```python
from build123d import *

# Parameters (mm, degrees)
SKETCH_1_W          = 42
SKETCH_1_H          = 76.3
EXTRUDE_1_DEPTH     = 20.5
FILLET_1_R          = 8
SHELL_1_T           = 2.3
CUT_EXTRUDE_START   = 2.2
SKETCH_3_W          = 37.8
SKETCH_3_H          = 71.7
CUT_EXTRUDE_1_DEPTH = 19.3
SKETCH_1_3_R        = 1.5
CUT_EXTRUDE_2_DEPTH = 21.5
SKETCH_4_W          = 1
SKETCH_4_H          = 76.3
EXTRUDE_2_DEPTH     = 20.5
CHAMFER1_SIZE       = 1.3


with BuildPart() as part:
    # Эскиз1 → Бобышка-Вытянуть1 (new body)
    with BuildSketch(Plane(origin=(0, 0, 0), x_dir=(1, 0, 0), z_dir=(0, 1, 0))):
        Rectangle(SKETCH_1_W, SKETCH_1_H)
    extrude(amount=EXTRUDE_1_DEPTH)

    # Скругление1
    fillet_1_edges = [part.edges().sort_by_distance(p)[0] for p in [
        (-21, 20.5, 0),
        (21, 20.5, 0),
    ]]
    fillet(fillet_1_edges, radius=FILLET_1_R)

    # Оболочка1 (no face opened: a closed hollow body)
    add(offset(amount=-SHELL_1_T, mode=Mode.PRIVATE), mode=Mode.SUBTRACT)

    # Эскиз3 → Вырез-Вытянуть1 (cut, through all)
    with BuildSketch(Plane(origin=(0, 0, 0), x_dir=(1, 0, 0), z_dir=(0, 1, 0)).offset(CUT_EXTRUDE_START)):
        Rectangle(SKETCH_3_W, SKETCH_3_H)
    extrude(amount=CUT_EXTRUDE_1_DEPTH, mode=Mode.SUBTRACT)

    # Эскиз1<3> → Вырез-Вытянуть2 (cut, through all)
    with BuildSketch(Plane(origin=(0, 0, 0), x_dir=(1, 0, 0), z_dir=(0, 1, 0))):
        with Locations((-10.5, 0)):
            Circle(SKETCH_1_3_R)
        with Locations((10.5, 0)):
            Circle(SKETCH_1_3_R)
    extrude(amount=CUT_EXTRUDE_2_DEPTH, mode=Mode.SUBTRACT)

    # Эскиз4 → Бобышка-Вытянуть2 (add)
    with BuildSketch(Plane(origin=(0, 0, 0), x_dir=(1, 0, 0), z_dir=(0, 1, 0))):
        Rectangle(SKETCH_4_W, SKETCH_4_H)
    extrude(amount=EXTRUDE_2_DEPTH)

    # Chamfer1
    chamfer1_edges = [part.edges().sort_by_distance(p)[0] for p in [
        (9, 2.2, 0),
        (-12, 2.2, 0),
    ]]
    chamfer(chamfer1_edges, length=CHAMFER1_SIZE)


solid = part.part
```
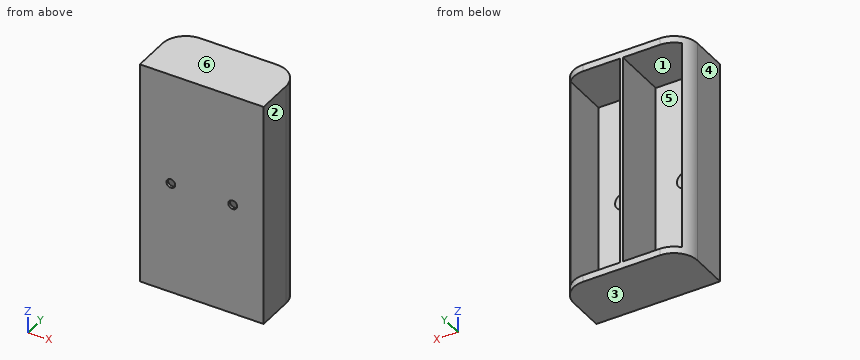
For this review, take the finished solid that the model builds, in its own axes (mm). Face numbers are marked on the shaded views. A direction names the side the tool comes from. Coordinates: 2 decimals unless noted, no trailing zeros. Write each loop counter-clockwise with the first axis right and the second up, starting at its lowest first coordinate (ties: lowest second). Pieces come first, ordered by that corner, then holes.
(1) The part is to be moulded in two halves that separate along Z. For the marked faces 3, 4, 5 and 6, say which applies: +Z half, -Z half, draft (parallel to the pull), parting line (faces both ways), or undercut.
(2) Add section C-C on x = 5.5. Give the boundary of the cut face in (y, z), then the cut area to 3 significant figures.
(3) Add section B-B on y = 5.25. Give the boundary of the cut face in (x, z).
(4) Tool access review of the marked faces 1 and 2: name each direction out of +Z, -Z, +X, -X, +Y, -Y from which nothing blocks a thin tool from reaching the whole face with its end or side.
(5) For pin 1 Ø8 at (x, z) = (7.5, 6.5) entering from -Y; pin 2 Ø4 at (y, z) = (16, 20.5) entering from -X; pin 3 Ø9 at (x, z) = (6.5, 15) entering from +Y; pin 4 Ø1 at (y, z) = (16, -6.5) entering from -X, all flat-tipped, find the tip position at first contact; note any pin that passes through.
(6) Wall thickness on probe 1 along X at (y, z) = (2.25, 30.5); probe 2 along X at (y, z) = (0.2, 0); probe 3 along Z at (x, y) = (10.5, 0.45): over which ranges is each line inside the solid? List them lowest first.
(7) Add section D-D on z = -19. Give the boundary of the cut face in (x, y).
(8) Add section A-A on x = 10.5. Give the boundary of the cut face in (y, z), then the cut area to 3 significant figures.
Answer sheet:
1. face 3: -Z half
1. face 4: draft
1. face 5: undercut
1. face 6: +Z half
2. outline: (0, -38.15) - (20.5, -38.15) - (20.5, -35.85) - (2.2, -35.85) - (2.2, 35.85) - (20.5, 35.85) - (20.5, 38.15) - (0, 38.15) - close
2. area: 252 mm2
3. outline: (-21, -38.15) - (21, -38.15) - (21, 38.15) - (-21, 38.15) - close; hole (-18.9, -35.85) - (-0.5, -35.85) - (-0.5, 35.85) - (-18.9, 35.85) - close; hole (0.5, -35.85) - (18.9, -35.85) - (18.9, 35.85) - (0.5, 35.85) - close
4. face 1: +Y
4. face 2: +Z, -Z, +X, +Y, -Y
5. pin 1: stops at y = 0
5. pin 2: stops at x = -20.86
5. pin 3: stops at y = 2.2
5. pin 4: stops at x = -20.42
6. probe 1: x = -21 to -18.9, -0.5 to 0.5, 18.9 to 21
6. probe 2: x = -21 to -12, -9 to 9, 12 to 21
6. probe 3: z = -38.15 to -1.5, 1.5 to 38.15
7. outline: (-21, 0) - (21, 0) - (21, 12.5) arc R8 ccw to (18.9, 17.9) - (18.9, 2.2) - (0.5, 2.2) - (0.5, 20.5) - (-0.5, 20.5) - (-0.5, 2.2) - (-18.9, 2.2) - (-18.9, 17.9) arc R8 ccw to (-21, 12.5) - close
8. outline: (0, -38.15) - (20.5, -38.15) - (20.5, -35.85) - (2.2, -35.85) - (2.2, -2.8) - (0.9, -1.5) - (0, -1.5) - close; (0, 1.5) - (0.9, 1.5) - (2.2, 2.8) - (2.2, 35.85) - (20.5, 35.85) - (20.5, 38.15) - (0, 38.15) - close
8. area: 244 mm2
